from build123d import *

# Parameters (mm, degrees)
FILLET1_R   = 0.1
HEX_2_DEPTH = 1.1


with BuildPart() as part:
    # BodySke → BaseBody (revolve)
    with BuildSketch(Plane.XY, mode=Mode.PRIVATE) as basebody_sk:
        Polygon((0, 0), (0, 3), (0.36, 3), (1.86, 1.5), (17.7195, 1.5), (18, 1.2195), (18, 0), align=None)
    revolve(basebody_sk.sketch.rotate(Axis((0, 0, 0), (1, 0, 0)), 90), axis=Axis((0, 0, 0), (1, 0, 0)))

    # Fillet1
    fillet1_edges = [part.edges().sort_by_distance(p)[0] for p in [
        (1.86, 0, -1.5),
    ]]
    fillet(fillet1_edges, radius=FILLET1_R)

    # Sketch2 → PreBroach (revolve, cut)
    with BuildSketch(Plane.XY, mode=Mode.PRIVATE) as prebroach_sk:
        Polygon((0, 1), (1.1, 1), (1.677350269, 0), (0, 0), align=None)
    revolve(prebroach_sk.sketch.rotate(Axis((0, 0, 0), (1, 0, 0)), 90), axis=Axis((0, 0, 0), (1, 0, 0)), mode=Mode.SUBTRACT)

    # Sketch3 → Hex 2 (cut)
    with BuildSketch(Plane.ZY):
        Polygon((-1, -0.577350269), (-1, 0.577350269), (0, 1.154700538), (1, 0.577350269), (1, -0.577350269), (0, -1.154700538), align=None)
    extrude(amount=-HEX_2_DEPTH, mode=Mode.SUBTRACT)


solid = part.part
Part model, mm, in its own coordinate system. A direction names the side the tool comes from. Coordinates: 2 decimals unless noted, no trailing zeros. Order: outer loops, then holes, each group sorted by start corner. A loop starts at its lowest first (then second) coordinate and runs counter-clockwise, first axis right, second up. Notation, with made-up numbers: M 10.5,13 L 31.5,13 A37 cw 31.5,49 Z; hole C 24.5,87.5 d5. An arc over 180 degrees is marked long. Use a Markdown table: item, result.
(1) Tool access for faces 1 (the flat face through (0.54, 0.87, 0.49)), 2 (the flat face through (18, 0, 0)), 3 (the cylindrical face through (9.92, -0.45, 1.43)): list every direction of +Z, -Z, +X, -X, +Y, -Y with a clear straight run to the whole face (end or side of a thin tool).
A:
| item | result |
|---|---|
| face 1 | -X |
| face 2 | +Z, -Z, +X, +Y, -Y |
| face 3 | +X |
(2) Cut at A-A on x = 8.75. Write the cut outline in (y, z), then the cut area to 3 significant figures.
A:
| item | result |
|---|---|
| outline | C 0,0 d3 |
| area | 7.07 mm^2 |
(3) Flat gauge pins, fed straight in: pin 1 (1.5 mm diameter, centred on x = 13.5, z = 0.5, fed in from -Y); pin 2 (2 mm diameter, centred on x = 8.5, y = -2, fed in from -Z); pin 3 (1.5 mm diameter, centred on x = 3, z = -1, fed in from +Y). Where does each tip first touch, or does it go through?
A:
| item | result |
|---|---|
| pin 1 | stops at y = -1.5 |
| pin 2 | stops at z = -1.12 |
| pin 3 | stops at y = 1.48 |
(4) Pull direction Z, two halves, no side cores. Call faces 4 (the flat face through (0.5, 0, -1)), 5 (the flat face through (0, 0, -1.3)), 6 (the cylindrical face through (0.18, -0.9, 2.86)): released by +Z, released by -Z, zero draft, split by the parting line, or undercut.
A:
| item | result |
|---|---|
| face 4 | undercut |
| face 5 | zero draft |
| face 6 | split by the parting line |
(5) Probe L1, parallel to Y at x = 13, z = -0.5; L2, parallel to X at y = -2.5, z = 0; L3, parallel to Y at x = 5, z = 0.75. List the from-to ranges inside material, lowest first.
A:
| item | result |
|---|---|
| L1 | y = -1.41 to 1.41 |
| L2 | x = 0 to 0.86 |
| L3 | y = -1.3 to 1.3 |
